```python
from build123d import *

# Parameters (mm, degrees)
SKETCH_1_R                       = 22.5
EXTRUDE_1_DEPTH                  = 2
EXTRUDE_2_DEPTH                  = 2
FILLET_1_R                       = 1
PATTERN_CIRCULAR_1_COUNT         = 12
FILLET_1_OF_PATTERN_CIRCULAR_1_R = 1
SKETCH_3_R                       = 4
CUT_EXTRUDE_1_DEPTH              = 2
SKETCH_4_R                       = 1
CUT_EXTRUDE_2_DEPTH              = 2
PATTERN_CIRCULAR_2_COUNT         = 3


with BuildPart() as part:
    # 草图1 → 凸台-拉伸1 (new body)
    with BuildSketch(Plane.XY):
        Circle(SKETCH_1_R)
    extrude(amount=EXTRUDE_1_DEPTH)

    # 草图2 → 凸台-拉伸2 (add)
    with BuildSketch(Plane.XY):
        with BuildLine():
            Line((0, 28.410934831), (-2.001953781, 22.410760386))
            ThreePointArc((-2.001953781, 22.410760386), (-0.000980777, 22.499999979), (2, 22.410934831))
            Line((2, 22.410934831), (0, 28.410934831))
        make_face()
    extrude_2 = extrude(amount=EXTRUDE_2_DEPTH)

    # 圆角1
    fillet_1_edges = [part.edges().sort_by_distance(p)[0] for p in [
        (0, 28.410934831, 1),
    ]]
    fillet(fillet_1_edges, radius=FILLET_1_R)

    # 阵列(圆周)1: 凸台-拉伸2 ×12 about axis
    pattern_circular_1_axis = Axis((0, 0, 0), (0, 0, 1))
    for i in range(1, PATTERN_CIRCULAR_1_COUNT):
        add(extrude_2.rotate(pattern_circular_1_axis, i * 360 / PATTERN_CIRCULAR_1_COUNT))

    # 圆角1 of 阵列(圆周)1
    fillet_1_of_pattern_circular_1_edges = [part.edges().sort_by_distance(p)[0] for p in [
        (-14.205467416, 24.604591309, 1),
        (-24.604591309, 14.205467416, 1),
        (-28.410934831, 0, 1),
        (-24.604591309, -14.205467416, 1),
        (-14.205467416, -24.604591309, 1),
        (0, -28.410934831, 1),
        (14.205467416, -24.604591309, 1),
        (24.604591309, -14.205467416, 1),
        (28.410934831, 0, 1),
        (24.604591309, 14.205467416, 1),
        (14.205467416, 24.604591309, 1),
    ]]
    fillet(fillet_1_of_pattern_circular_1_edges, radius=FILLET_1_OF_PATTERN_CIRCULAR_1_R)

    # 草图3 → 切除-拉伸1 (cut)
    with BuildSketch(Plane.XY.offset(2)):
        Circle(SKETCH_3_R)
    extrude(amount=-CUT_EXTRUDE_1_DEPTH, mode=Mode.SUBTRACT)

    # 草图4 → 切除-拉伸2 (cut)
    with BuildSketch(Plane.XY.offset(2)):
        with Locations((0, 14)):
            Circle(SKETCH_4_R)
    cut_extrude_2 = extrude(amount=-CUT_EXTRUDE_2_DEPTH, mode=Mode.SUBTRACT)

    # 阵列(圆周)2: 切除-拉伸2 ×3 about axis
    pattern_circular_2_axis = Axis((0, 0, 0), (0, 0, 1))
    for i in range(1, PATTERN_CIRCULAR_2_COUNT):
        add(cut_extrude_2.rotate(pattern_circular_2_axis, i * 360 / PATTERN_CIRCULAR_2_COUNT), mode=Mode.SUBTRACT)


solid = part.part
```
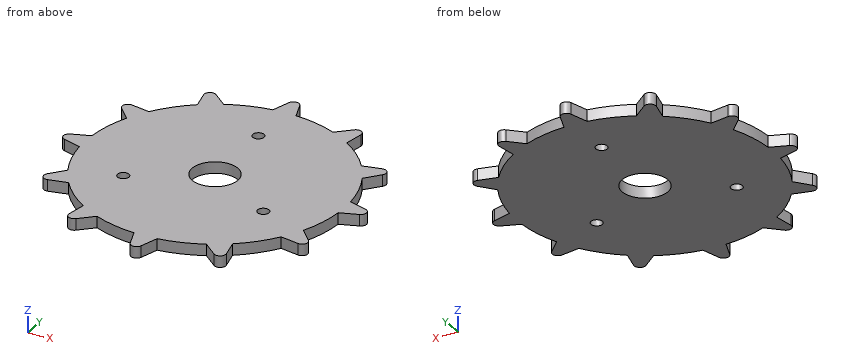
Verification items for the finished model (mm, model axes). Round coordinates to 2 decimals unless told otherwise and drop trailing zeros. Order: outer loops, then holes, each group sorted by start corner. A loop starts at its lowest first (then second) coordinate and runs counter-clockwise, first axis right, second up.
1) Cross-section at D-D, the plane x = 16.5. Record the cut outline in (y, z).
Geometry says:
outline: (-15.3, 0) - (15.3, 0) - (15.3, 2) - (-15.3, 2) - close
2) Cross-section at B-B, the plane y = -7. Record the cut outline in (x, z).
Geometry says:
outline: (-21.38, 0) - (-13.12, 0) - (-13.12, 2) - (-21.38, 2) - close; (-11.12, 0) - (11.12, 0) - (11.12, 2) - (-11.12, 2) - close; (13.12, 0) - (21.38, 0) - (21.38, 2) - (13.12, 2) - close
3) Material ranges on line 1 (Y direction, x = 0, z = 1); line 2 (Y direction, x = 22.5, z = 0.5); line 3 (Y direction, x = -12.5, z = 0.8), recorded low to high.
Geometry says:
line 1: y = -26.25 to -4, 4 to 13, 15 to 26.25
line 2: y = -13.4 to -11.83, -1.97 to 1.97, 11.83 to 13.4
line 3: y = -22.86 to -7.93, -6.07 to 22.86
4) Cross-section at A-A, the plane x = 0. Record the cut outline in (y, z), plus the area to 3 significant figures.
Geometry says:
outline: (-26.25, 0) - (-4, 0) - (-4, 2) - (-26.25, 2) - close; (4, 0) - (13, 0) - (13, 2) - (4, 2) - close; (15, 0) - (26.25, 0) - (26.25, 2) - (15, 2) - close
area: 85.0 mm2
5) Cross-section at C-C, the plane z = 0.85. Give the number of separate pieces and of enclosed holes in the cut face, plus the area to 3 significant figures.
Geometry says:
separate pieces: 1
enclosed holes: 4
area: 1,650 mm2
